The model under review builds one solid part; all positions refer to its coordinate system, in mm. Face numbers are marked on the shaded views. Coordinates: 2 decimals unless noted, no trailing zeros. Put each result on its own line as item: value.
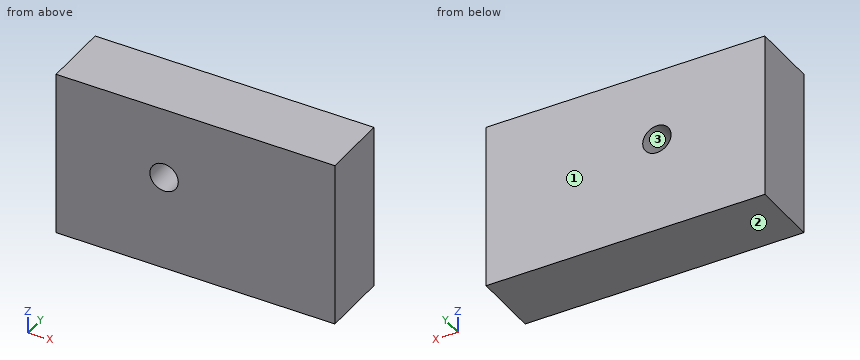
from build123d import *

# Parameters (mm, degrees)
SKETCH1_W                 = 41.295636026
SKETCH1_H                 = 24.657103064
BOSS_EXTRUDE1_DEPTH       = 10
M5X0_8_TAPPED_HOLE1_D     = 4.2
M5X0_8_TAPPED_HOLE1_DEPTH = 14
M5X0_8_TAPPED_HOLE1_TIP   = 1.2618073


with BuildPart() as part:
    # Sketch1 → Boss-Extrude1 (new body)
    with BuildSketch(Plane(origin=(0, 0, 0), x_dir=(1, 0, 0), z_dir=(0, 1, 0))):
        with Locations((1.60371402, 1.202785515)):
            Rectangle(SKETCH1_W, SKETCH1_H)
    extrude(amount=-BOSS_EXTRUDE1_DEPTH)

    # M5x0.8 Tapped Hole1
    with Locations(Plane(origin=(0, 0, 0), x_dir=(-1, 0, 0), z_dir=(0, 1, 0))):
        with Locations((3.044035574, 0.569159987)):
            Hole(M5X0_8_TAPPED_HOLE1_D / 2, depth=M5X0_8_TAPPED_HOLE1_DEPTH)
            with Locations((0, 0, -(M5X0_8_TAPPED_HOLE1_DEPTH + M5X0_8_TAPPED_HOLE1_TIP / 2))):  # 118° drill point
                Cone(0, M5X0_8_TAPPED_HOLE1_D / 2, M5X0_8_TAPPED_HOLE1_TIP, mode=Mode.SUBTRACT)


solid = part.part
1. For pin 1 Ø12 at (x, z) = (-11, -6.5) entering from +Y; pin 2 Ø3.5 at (x, z) = (-3.04, 0.57) entering from +Y, all flat-tipped, find the tip position at first contact; note any pin that passes through.
Determined:
pin 1: stops at y = 0
pin 2: passes through
2. The part is to be moulded in two halves that separate along Z. For the marked faces 1, 2 and 3, say which applies: +Z half, -Z half, draft (parallel to the pull), parting line (faces both ways), or undercut.
Determined:
face 1: draft
face 2: -Z half
face 3: undercut
3. To check wall thickness, follow probe 1 along X at (y, z) = (-7.75, -1.25). State the ranges of the line that lie inside material, in increasing order.
Determined:
probe 1: x = -19.04 to -4.09, -1.99 to 22.25
